Here's the drawing with two shaded views (mm, measured from the low corner). I have some questions. Round coordinates to 2 decimals unless told otherwise and drop trailing zeros. Order: outer loops, then holes, each group sorted by start corner. A loop starts at its lowest first (then second) coordinate and runs counter-clockwise, first axis right, second up. Notation, with made-up numbers: (-25.5, -25.5) -> (20.5, -25.5) arc R34 cw to (20.5, 9.5) -> close; hole circle Ø2 at (74.5, -21.5). An arc over 180 degrees is marked (long way). Answer in a Markdown table with one row per item.
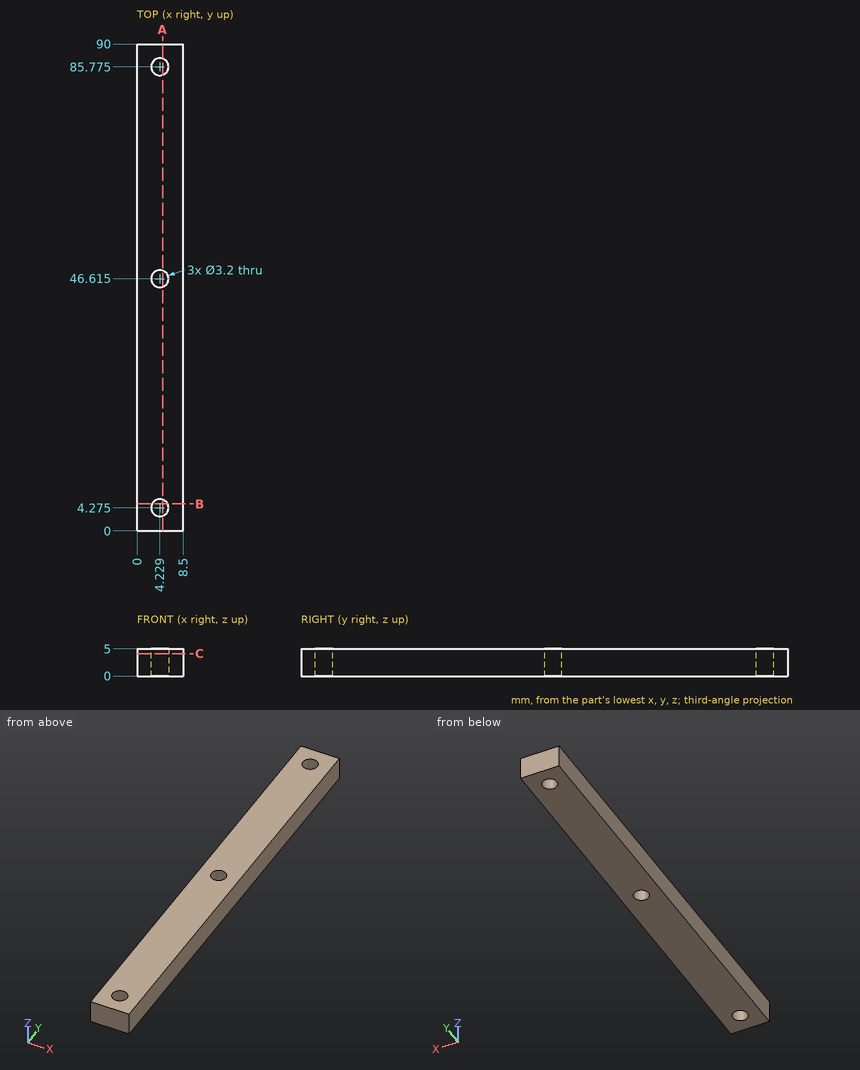
1. Please list where these lines run through material, in increasing order: line 1 along Y through (x, z) = (5, 1.55); line 2 along Y through (x, z) = (3, 2.6); line 3 along X through (y, z) = (85.5, 1).
Numbers:
| item | result |
|---|---|
| line 1 | y = 0 to 2.87, 5.68 to 45.21, 48.02 to 84.37, 87.18 to 90 |
| line 2 | y = 0 to 3.25, 5.3 to 45.59, 47.64 to 84.75, 86.8 to 90 |
| line 3 | x = 0 to 2.65, 5.81 to 8.5 |
2. Suppose I cut it at B-B on y = 5. Write out the boundary of the cut face in (x, z), then the cut area to 3 significant figures.
Numbers:
| item | result |
|---|---|
| outline | (0, 0) -> (2.8, 0) -> (2.8, 5) -> (0, 5) -> close; (5.66, 0) -> (8.5, 0) -> (8.5, 5) -> (5.66, 5) -> close |
| area | 28.2 mm2 |
3. Suppose I cut it at C-C on z = 4.15. Write out the boundary of the cut face in (x, y) (3 decimals).
Numbers:
| item | result |
|---|---|
| outline | (0, 0) -> (8.5, 0) -> (8.5, 90) -> (0, 90) -> close; hole circle Ø3.2 at (4.229, 4.275); hole circle Ø3.2 at (4.229, 46.615); hole circle Ø3.2 at (4.229, 85.775) |
4. For pin 1 Ø1.9 at (x, y) = (4.23, 46.61) entering from -Z (1 decimal); pin 2 Ø4 at (x, y) = (4.23, 4.27) entering from +Z, each with a flat end and sliding along its axis, tell me the tip position at first contact or that it passes through.
Numbers:
| item | result |
|---|---|
| pin 1 | passes through |
| pin 2 | stops at z = 5 |
5. Suppose I cut it at A-A on x = 4.75. Write out the boundary of the cut face in (y, z), then the cut area to 3 significant figures.
Numbers:
| item | result |
|---|---|
| outline | (0, 0) -> (2.76, 0) -> (2.76, 5) -> (0, 5) -> close; (5.79, 0) -> (45.1, 0) -> (45.1, 5) -> (5.79, 5) -> close; (48.13, 0) -> (84.26, 0) -> (84.26, 5) -> (48.13, 5) -> close; (87.29, 0) -> (90, 0) -> (90, 5) -> (87.29, 5) -> close |
| area | 405 mm2 |
